Source: CAD feature listing. Evaluate the final solid. Frame: model axes, mm. A direction names the side the tool comes from. Round coordinates to 2 decimals unless told otherwise and drop trailing zeros. Write each loop counter-clockwise with the first axis right and the second up, starting at its lowest first coordinate (ties: lowest second). Pieces come first, ordered by that corner, then holes. Notation, with made-up numbers: (73.5, 36) -> (77.5, 36) arc R13 ccw to (77.5, 52) -> close; hole circle Ø9 at (60.25, -14). An arc over 180 degrees is marked (long way). Put each result on its own line as item: value.
```python
from build123d import *

# Parameters (mm, degrees)
F0_R          = 4
F0_R_2        = 2.5
F1_DEPTH      = 0.7
F2_R          = 3.3
F2_R_2        = 2.5
F3_DEPTH      = 1
F4_R          = 4
F4_R_2        = 2.7082847247
F5_DEPTH      = 0.7
F9_ANGLE_BACK = 20
F9_ANGLE      = 40


with BuildPart() as f1:
    # F0 (on Top) → F1 (new body)
    with BuildSketch(Plane.XY):
        Circle(F0_R)
        Circle(F0_R_2, mode=Mode.SUBTRACT)
    extrude(amount=F1_DEPTH)

    # F2 (on face) → F3 (join)
    with BuildSketch(Plane.XY.offset(0.7)):
        Circle(F2_R)
        Circle(F2_R_2, mode=Mode.SUBTRACT)
    extrude(amount=F3_DEPTH)

    # F4 (on face) → F5 (join)
    with BuildSketch(Plane.XY.offset(1.7)):
        Circle(F4_R)
        Circle(F4_R_2, mode=Mode.SUBTRACT)
    extrude(amount=F5_DEPTH)

    # F6 (on Right) → F7 (revolve)
    with BuildSketch(Plane.YZ):
        Polygon((-4, 1.7), (-4, 2.4), (-4.7, 2.4), align=None)
        Polygon((-3.3, 1.7), (-4, 1.7), (-3.3, 1.4059272362), align=None)
    revolve(axis=Axis((0, 0, 2.4), (0, 0, 1)))

    # F8 (on Right) → F9 (revolve)
    with BuildSketch(Plane.YZ, mode=Mode.PRIVATE) as f9_sk:
        with BuildLine():
            add(Edge.make_bspline(
                [(-3.3, 1.4059272362), (-6.0468855435, 1.441646311), (-6.2736891755, 2.9814417815), (-4.7089018779, 13.0197805627), (-4.5280783622, 13.8493191708), (-3.9012755567, 14.3429894387), (-3.5414669526, 13.2946596808), (-4.3496219383, 12.8327032699), (-5.097212262, 2.7888434187), (-4.9865280125, 2.7266615906), (-4.7, 2.4)],
                knots=[0, 0, 0, 0, 0.1500571493, 0.3998382837, 0.4758785019, 0.5317203727, 0.5995110586, 0.6784641499, 0.9265496454, 1, 1, 1, 1], degree=3))
            Line((-3.3, 1.4059272362), (-4, 1.7))
            Line((-4, 1.7), (-4.7, 2.4))
        make_face()
    revolve(f9_sk.sketch.rotate(Axis((0, 0, 2.4), (0, 0, 1)), -F9_ANGLE_BACK), axis=Axis((0, 0, 2.4), (0, 0, 1)), revolution_arc=F9_ANGLE)

    # F10: F1 across plane


with BuildPart() as f1_1:
    add(f1.part)
    add(f1.part.mirror(Plane.XZ))


solid = f1_1.part
```
Q1. Draft query along Z for faces 6 (the flat face through (-2, 3, 0.7)), 7 (the conical face through (-3.489, 0.06, 1.486)), 8 (the flat face through (2, 2, 0)), 9 (the cylindrical face through (-0.867, -3.905, 0.345)). Return one class per face: +Z half, -Z half, draft (parallel to the pull), parting line (faces both ways), or undercut.
Ans:
face 6: undercut
face 7: undercut
face 8: -Z half
face 9: draft
Q2. Cut plane A-A on y = 0. Output: boundary loops of the cut face in (x, z), and give its area (3 significant figures).
Ans:
outline: (-4.7, 2.4) -> (-4, 1.7) -> (-3.3, 1.41) -> (-3.3, 0.7) -> (-4, 0.7) -> (-4, 0) -> (-2.5, 0) -> (-2.5, 1.7) -> (-2.71, 1.7) -> (-2.71, 2.4) -> close; (2.5, 0) -> (4, 0) -> (4, 0.7) -> (3.3, 0.7) -> (3.3, 1.41) -> (4, 1.7) -> (4.7, 2.4) -> (2.71, 2.4) -> (2.71, 1.7) -> (2.5, 1.7) -> close
area: 6.20 mm^2
Q3. Material intervals for line 1 (Y direction, x = 0, z = 1.2); line 2 (Z direction, x = -0.25, y = -3.5); line 3 (Z direction, x = 2.5, y = -1.5), sorted ascending. Write a range as [from, to].
Ans:
line 1: y = [-3.3, -2.5], [2.5, 3.3]
line 2: z = [0, 0.7], [1.41, 2.4]
line 3: z = [0, 2.4]
Q4. Reachability of faces 1 (the cylindrical face through (2.5, -1.04, 2.05)), 2 (the conical face through (3.489, -0.06, 1.486)), 3 (the cylindrical face through (3.15, 0.99, 1.05)), 4 (the conical face through (-4.11, 0.07, 1.81)), 5 (the cylindrical face through (-0.54, -2.44, 0.84)) from +Z, -Z, +X, -X, +Y, -Y: full face, straight path, thin tool, end or side. Return the list, or none.
Ans:
face 1: +Z
face 2: +X
face 3: none
face 4: -Z, -X
face 5: +Z, -Z
Q5. Pin query (flat end, axial travel): pin 1 (5 mm diameter, centred on x = -2.5, z = 8, fed in from +Y); pin 2 (4 mm diameter, centred on x = 0.5, y = -1, fed in from +Z); pin 3 (1 mm diameter, centred on x = -1.5, z = 8.5, fed in from -Y); pin 4 (3 mm diameter, centred on x = 0, y = 0, fed in from -Z). Return the tip coordinate at first contact, or that it passes through.
Ans:
pin 1: stops at y = 5.65
pin 2: stops at z = 2.4
pin 3: stops at y = -5.32
pin 4: passes through
